CAD build for the part. Positions are in the model's coordinates, mm. A direction names the side the tool comes from. Round coordinates to 2 decimals unless told otherwise and drop trailing zeros. Write each loop counter-clockwise with the first axis right and the second up, starting at its lowest first coordinate (ties: lowest second). Pieces come first, ordered by that corner, then holes. Notation, with made-up numbers: (74.5, 25) -> (106.5, 25) arc R20 cw to (106.5, 35) -> close; hole circle Ø9 at (-23, 28.25). An arc over 180 degrees is marked (long way). Answer in a Markdown table with one row per item. Add a question column.
```python
from build123d import *

# Parameters (mm, degrees)
F0_W     = 53.5
F0_H     = 1.5
F0_W_2   = 1.5
F1_DEPTH = 10
F2_R     = 1
F3_R     = 1


with BuildPart() as f1:
    # F0 (on Front) → F1 (new body)
    with BuildSketch(Plane.XZ):
        with Locations((26.75, -0.75)):
            Rectangle(F0_W, F0_H)
        Polygon((0, 9), (0, 0), (53.5, 0), align=None)
        with Locations((-0.75, -0.75)):
            Rectangle(F0_W_2, F0_H)
        Polygon((53.5, 11), (53.5, 0), (53.5, -1.5), (54.999999, -1.5), (54.999999, 18.5), (53.5, 18.5), align=None)
        Polygon((-1.5, 0), (0, 0), (0, 9), (0, 17), (53.5, 11), (53.5, 18.5), (-1.500001, 18.5), align=None)
    extrude(amount=F1_DEPTH)

    # F2
    f2_edges = [f1.edges().sort_by_distance(p)[0] for p in [
        (54.999999, -10, 8.5),
        (26.749999, -10, 18.5),
        (26.75, -10, -1.5),
        (-1.5, -10, 9.25),
        (-1.5, -10, -0.75),
        (-1.5, -5, -1.5),
        (-1.500001, -5, 18.5),
        (54.999999, -5, 18.5),
        (54.999999, -5, -1.5),
    ]]
    fillet(f2_edges, radius=F2_R)

    # F3
    f3_edges = [f1.edges().sort_by_distance(p)[0] for p in [
        (0, -5, 17),
        (0, -5, 9),
        (53.5, -5, 11),
        (53.5, -5, 0),
    ]]
    fillet(f3_edges, radius=F3_R)


solid = f1.part
```
Item 1: Saw through at A-A on z = 14. Give the cut face in (x, y).
Item 2: Two-plate mould, pull along X, no slides. Class faces 3 (the cylindrical face through (54.715, -9.699, 8.626)), 4 (the cylindrical face through (53.24, -5.07, 10.78)), 5 (the flat face through (27, -4, 18.5)): +X half, -X half, draft (parallel to the pull), parting line (faces both ways), or undercut.
Item 3: Pin check, flat tip, straight feed: pin 1 (10 mm diameter, centred on x = 10.5, z = 8.5, fed in from -Y). Stop position of the tip, or through.
Item 4: Tool access for faces 1 (the cylindrical face through (53.136, -5.07, 0.411)), 2 (the flat face through (55, -4, 8)): list every direction of +Z, -Z, +X, -X, +Y, -Y with a clear straight run to the whole face (end or side of a thin tool).
Item 5: Saw through at B-B on y = -5.25. Give the cut face in (x, z).
Item 6: Saw through at C-C on x = 17. Give the cut face in (y, z), then the cut area to 3 significant figures.
Item 7: Drill centre lines: probe 1 along X at (y, z) = (-4, 10); probe 2 along Z at (x, y) = (9.5, -6); probe 3 along Z at (x, y) = (41, -7). Where is each one in solid material? Low to high.
Recorded:
| question | item | result |
|---|---|---|
| 1 | outline | (-1.5, -9) arc R1 ccw to (-0.5, -10) -> (0, -10) -> (0, 0) -> (-1.5, 0) -> close; (26.75, -10) -> (54, -10) arc R1 ccw to (55, -9) -> (55, 0) -> (26.75, 0) -> close |
| 2 | face 3 | +X half |
| 2 | face 4 | undercut |
| 2 | face 5 | draft |
| 3 | pin 1 | y = -10 |
| 4 | face 1 | +Y, -Y |
| 4 | face 2 | +Z, -Z, +X, +Y, -Y |
| 5 | outline | (-1.5, -0.5) arc R1 ccw to (-0.5, -1.5) -> (54, -1.5) arc R1 ccw to (55, -0.5) -> (55, 17.5) arc R1 ccw to (54, 18.5) -> (-0.5, 18.5) arc R1 ccw to (-1.5, 17.5) -> close; hole (0, 9.85) arc R1 ccw to (0.83, 8.86) -> (52.33, 0.2) arc R1 ccw to (53.5, 1.18) -> (53.5, 10.11) arc R1 ccw to (52.61, 11.1) -> (1.11, 16.88) arc R1 ccw to (0, 15.88) -> close |
| 6 | outline | (-10, -0.5) arc R1 ccw to (-9, -1.5) -> (0, -1.5) -> (0, 6.14) -> (-10, 6.14) -> close; (-10, 15.09) -> (0, 15.09) -> (0, 18.5) -> (-9, 18.5) arc R1 ccw to (-10, 17.5) -> close |
| 6 | area | 110 mm2 |
| 7 | probe 1 | -1.5 to 0, 53.5 to 55 |
| 7 | probe 2 | -1.5 to 7.4, 15.93 to 18.5 |
| 7 | probe 3 | -1.5 to 2.1, 12.4 to 18.5 |
